Answer from the drawing. Dimensions are ordinates in mm from the lowest x, y and z of the part. Round coordinates to 2 decimals unless told otherwise and drop trailing zeros. Loops run counter-clockwise (first coordinate to the right, second up) from the corner with the lowest first, then second, coordinate; pieces in that order, holes last.
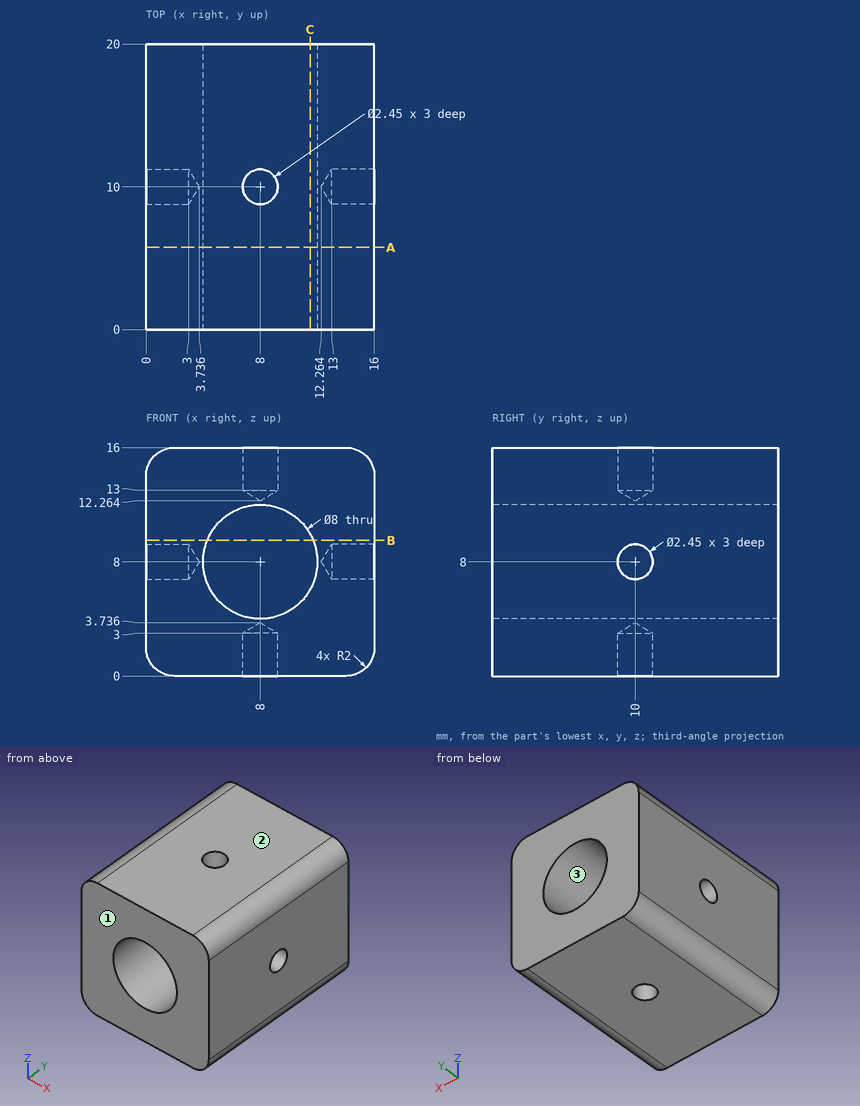
Item 1: Straight lines are drawn through the part: line 1 (Y direction, x = 8, z = 15.05) (3 decimals); line 2 (Z direction, x = 8, y = 15); line 3 (X direction, y = 10, z = 0.7) (3 decimals). For each, find the intervals that lie inside material, in ascending order.
Item 2: Section B-B, the plane z = 9.5 is taken. Give the vertices of the cut face in (x, y).
Item 3: Determine the mould class of the marked faces 1, 2 and 3 for opening direction Z: pulls with the +Z half, pulls with the -Z half, needs draft (parallel to the pull), parting line crosses it, or undercut.
Item 4: Each of these flat-tipped pins is pushed along its axis until it touches: P1, Ø2, axis at y = 10, z = 8, coming from the -X side; P2, Ø2, axis at x = 8, y = 10, coming from the +Z side. Where does it stop, or does it pass through?
Item 5: Section C-C, the plane x = 11.5 is taken. Give the vertices of the cut face in (y, z).
Item 6: Section A-A, the plane y = 5.75 is taken. Give the vertices of the cut face in (x, z).
Answer below:
1. line 1: y = 0 to 8.775, 11.225 to 20
1. line 2: z = 0 to 4, 12 to 16
1. line 3: x = 0.48 to 6.775, 9.225 to 15.52
2. outline: (0, 0) - (4.29, 0) - (4.29, 20) - (0, 20) - close; (11.71, 0) - (16, 0) - (16, 20) - (11.71, 20) - close
3. face 1: needs draft
3. face 2: pulls with the +Z half
3. face 3: undercut
4. P1: stops at x = 3.14
4. P2: stops at z = 12.86
5. outline: (0, 0) - (20, 0) - (20, 6.06) - (0, 6.06) - close; (0, 9.94) - (20, 9.94) - (20, 16) - (0, 16) - close
6. outline: (0, 2) arc R2 ccw to (2, 0) - (14, 0) arc R2 ccw to (16, 2) - (16, 14) arc R2 ccw to (14, 16) - (2, 16) arc R2 ccw to (0, 14) - close; hole circle Ø8 at (8, 8)
